Here's the drawing with two shaded views (mm, measured from the low corner). I have some questions. A direction names the side the tool comes from. Give positions to 0.01 mm unless a question says otherwise; leave off trailing zeros. Write each loop counter-clockwise with the first axis right and the second up, starting at its lowest first coordinate (ties: lowest second). Pieces come first, ordered by that corner, then holes. Notation, with made-up numbers: M 0,16.5 L 37,16.5 A18 cw 37,43.5 Z; hole C 67,-17 d1. An arc over 180 degrees is marked long. Answer as CSV lines item,"result". Start each with the question number.
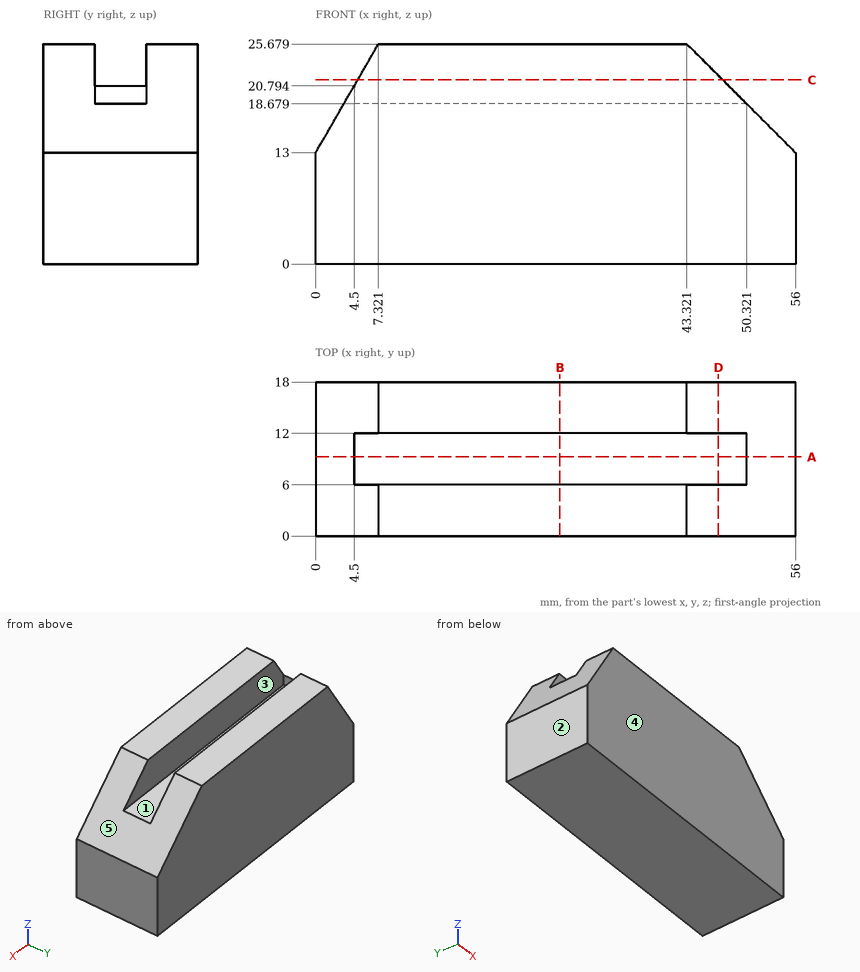
1. On a 3-axis mill with a long thin cutter (end or side, diameter ignored), from which of +Z, -Z, +X, -X, +Y, -Y can I reach the whole of each face in a straight line? I mean the marked faces 1 and 2. Say none if no direction works.
2. Imagine slicing it at D-D, the plane x = 47. Please give me the cut outline in (y, z).
3. Thinking about a two-plate mould opening in Y: for the marked faces 3, 4 and 5, which applies, pulls with the +Y half, pulls with the -Y half, needs draft (parallel to the pull), parting line crosses it, or undercut?
4. Imagine slicing it at C-C, the plane z = 21.5. Please give me the cut outline in (x, y).
5. Imagine slicing it at B-B, the plane x = 28.5. Please give me the cut outline in (y, z).
6. Will these pins go through, and if not, where does the flat tip stop? P1, Ø3, axis at y = 11, z = 20.5, coming from the -X side (1 decimal); P2, Ø4, axis at y = 2, z = 16.5, coming from the +X side; P3, Ø2.5, axis at y = 10, z = 19.5, coming from the +X side.
7. Please list where these lines run through material, in increasing order: line 1 (Y direction, x = 26, z = 18.75); line 2 (Z direction, x = 36, y = 10); line 3 (Z direction, x = 48, y = 3.75).
8. Imagine slicing it at A-A, the plane y = 9.25. Please give me the cut outline in (x, z) (1 decimal), plus the area to 3 significant figures.
Solutions:
1,face 1,"+Z, +X"
1,face 2,"+Z, -Z, -X, +Y, -Y"
2,outline,"M 0,0 L 18,0 L 18,22 L 12,22 L 12,18.68 L 6,18.68 L 6,22 L 0,22 Z"
3,face 3,"undercut"
3,face 4,"pulls with the -Y half"
3,face 5,"needs draft"
4,outline,"M 4.91,0 L 47.5,0 L 47.5,6 L 4.91,6 Z; M 4.91,12 L 47.5,12 L 47.5,18 L 4.91,18 Z"
5,outline,"M 0,0 L 18,0 L 18,25.68 L 12,25.68 L 12,18.68 L 6,18.68 L 6,25.68 L 0,25.68 Z"
6,P1,"x = 3.5"
6,P2,"x = 54.5"
6,P3,"x = 50.75"
7,line 1,"0 to 6, 12 to 18"
7,line 2,"0 to 18.68"
7,line 3,"0 to 21"
8,outline,"M 0,0 L 56,0 L 56,13 L 50.3,18.7 L 4.5,18.7 L 4.5,20.8 L 0,13 Z"
8,area,"1,020 mm²"
